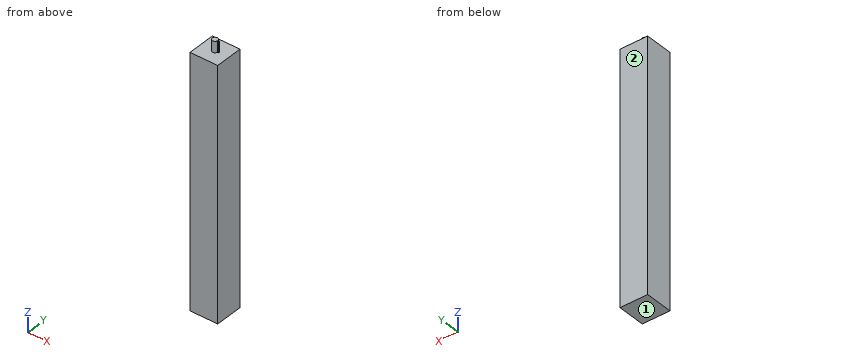
```python
from build123d import *

# Parameters (mm, degrees)
F1_DEPTH = 5
F3_DEPTH = 2
F4_DEPTH = 2
F5_R     = 0.01


with BuildPart() as f1:
    # F0 (on Front) → F1 (new body)
    with BuildSketch(Plane.XZ):
        Polygon((-2.5, 45), (-2.5, 0), (2.5, 0), (2.5, 45), (0, 45), align=None)
    extrude(amount=F1_DEPTH)

    # F2 (on face) → F3 (join)
    with BuildSketch(Plane.XY.offset(45)):
        with BuildLine():
            ThreePointArc((0.489898, -2.6), (0.497468, -2.550254), (0.5, -2.5))
            ThreePointArc((0.5, -2.5), (0.497468, -2.449746), (0.489898, -2.4))
            ThreePointArc((0.489898, -2.4), (-0.5, -2.5), (0.489898, -2.6))
        make_face()
    extrude(amount=F3_DEPTH)

    # F2 (on face) → F4 (join, through all)
    with BuildSketch(Plane.XY.offset(45)):
        with BuildLine():
            ThreePointArc((0.489898, -2.4), (0.497468, -2.449746), (0.5, -2.5))
            ThreePointArc((0.5, -2.5), (0.497468, -2.550254), (0.489898, -2.6))
            Line((0.489898, -2.6), (0.689898, -2.6))
            Line((0.689898, -2.6), (0.689898, -2.5))
            Line((0.689898, -2.5), (0.689898, -2.4))
            Line((0.689898, -2.4), (0.489898, -2.4))
        make_face()
    extrude(amount=F4_DEPTH)

    # F5
    f5_edges = [f1.edges().sort_by_distance(p)[0] for p in [
        (0.589898, -2.6, 47),
        (0.689898, -2.5, 47),
        (0.589898, -2.4, 47),
        (-0.5, -2.5, 47),
    ]]
    fillet(f5_edges, radius=F5_R)


solid = f1.part
```
CAD build for the part. Positions are in the model's coordinates, mm. Face numbers are marked on the shaded views. Coordinates: 2 decimals unless noted, no trailing zeros. Order: outer loops, then holes, each group sorted by start corner. A loop starts at its lowest first (then second) coordinate and runs counter-clockwise, first axis right, second up. Notation, with made-up numbers: M -38.75,71 L -12.75,71 A17 cw -12.75,103 Z; hole C 54,83 d3. An arc over 180 degrees is marked long. Write each question's results on one line, items separated by ' | '. Start each with the question number.
Q1. Cut at B-B (y = -1). List the corners of the cut face in (x, z), then the cut area to 3 significant figures.
Q2. Cut at A-A (x = 1.85). List the corners of the cut face in (y, z), then the cut area to 3 significant figures.
Q3. Drill centre line: probe 1 along Z at (x, y) = (0.55, -1.05). Where is it in solid material? Low to high. Write a range as from..to.
Q4. Pull direction Z, two halves, no side cores. Call the marked faces 1 and 2: +Z half, -Z half, draft (parallel to the pull), parting line (faces both ways), or undercut.
Found:
1) outline: M -2.5,0 L 2.5,0 L 2.5,45 L -2.5,45 Z | area: 225 mm²
2) outline: M -5,0 L 0,0 L 0,45 L -5,45 Z | area: 225 mm²
3) probe 1: 0..45
4) face 1: -Z half | face 2: draft
